Can you work these out from the model? Positions are in its coordinate system, mm. A direction names the side the tool comes from. Give positions to 0.01 mm unless a question says otherwise; leave off trailing zeros. Order: outer loops, then holes, each group sorted by start corner. A loop starts at its lowest first (then second) coordinate and runs counter-clockwise, first axis right, second up. Notation, with made-up numbers: (1.5, -24) - (36.5, -24) arc R32 ccw to (36.5, 11) - close; hole circle Ø11 at (77, -7). An arc over 180 degrees is marked (long way). Answer as a JSON object with one key per item and string values.
```python
from build123d import *

# Parameters (mm, degrees)
BOSS_EXTRUDE1_DEPTH = 438.15
CUT_EXTRUDE1_DEPTH  = 438.15


with BuildPart() as part:
    # Sketch2 → Boss-Extrude1 (new body)
    with BuildSketch(Plane(origin=(0, 0, 0), x_dir=(1, 0, 0), z_dir=(0, 1, 0))):
        Polygon((0, 0), (3.175, 0), (3.175, 22.225), (14.2875, 22.225), (14.2875, 25.4), (-11.1125, 25.4), (-11.1125, 22.225), (0, 22.225), align=None)
    extrude(amount=BOSS_EXTRUDE1_DEPTH)

    # Sketch4 → Cut-Extrude1 (cut)
    with BuildSketch(Plane(origin=(3.175, 0, 0), x_dir=(0, 0, -1), z_dir=(1, 0, 0))):
        Polygon((22.225, 0), (0, 45.568002879), (0, 0), align=None)
        Polygon((22.225, 438.15), (0, 427.310143219), (0, 438.15), align=None)
    extrude(amount=-CUT_EXTRUDE1_DEPTH, mode=Mode.SUBTRACT)


solid = part.part
```
Q1. If we section it at C-C, the plane z = -15.5: Please give me the cut outline in (x, y) (3 decimals), then the cut area to 3 significant figures.
Recorded:
{"outline": "(0, 13.788) - (3.175, 13.788) - (3.175, 434.87) - (0, 434.87) - close", "area": "1,340 mm^2"}
Q2. If we section it at B-B, the plane x = 10: Please give me the cut outline in (y, z) (3 decimals).
Recorded:
{"outline": "(0, -25.4) - (438.15, -25.4) - (438.15, -22.225) - (0, -22.225) - close"}
Q3. If we section it at A-A, the plane y = 313.5: Please give me the cut outline in (x, z) (1 decimal).
Recorded:
{"outline": "(-11.1, -25.4) - (14.3, -25.4) - (14.3, -22.2) - (3.2, -22.2) - (3.2, 0) - (0, 0) - (0, -22.2) - (-11.1, -22.2) - close"}
Q4. I need wall thicknesses on L1, parallel to X at y = 407, z = -9 (3 decimals); L2, parallel to Z at x = -6.25, y = 140.5 (3 decimals); L3, parallel to Y at x = 2, z = -2.5. Which ranges of each line are inside material? Lowest first, please.
Recorded:
{"L1": "x = 0 to 3.175", "L2": "z = -25.4 to -22.225", "L3": "y = 40.44 to 428.53"}
Q5. Which directions (+Z, -Z, +X, -X, +Y, -Y) give clear straight access to the entire face, cutting with the end or side of a thin tool? Please do faces 1 (the face through (-6, 216, -22.225)), 2 (the face through (9, 216, -22.225)), 3 (the face through (1.61, 432.806, -11.268)).
Recorded:
{"face 1": "+Z, -X, +Y, -Y", "face 2": "+Z, +X, +Y, -Y", "face 3": "+Z, +X, -X, +Y"}
Q6. I'm going to push flat-ended pins straight in: pin 1 Ø8 at (x, z) = (9, -3.5) entering from +Y; pin 2 Ø10 at (x, y) = (-7, 90) entering from +Z (3 decimals); pin 3 Ø5 at (y, z) = (121.5, -3.5) entering from -X. Where does each tip first touch, or does it pass through?
Recorded:
{"pin 1": "passes through", "pin 2": "stops at z = -22.225", "pin 3": "stops at x = 0"}
